The drawing under review shows one solid part. Ordinate dimensions are in mm from its lowest x, y, z. A direction names the side the tool comes from. Round coordinates to 2 decimals unless told otherwise and drop trailing zeros. Order: outer loops, then holes, each group sorted by start corner. A loop starts at its lowest first (then second) coordinate and runs counter-clockwise, first axis right, second up. Notation, with made-up numbers: (14, 16) - (25, 16) arc R30 ccw to (25, 53) - close; hole circle Ø3 at (22.5, 33.5). An arc over 180 degrees is marked (long way). One line per question, with ' | ' between items.
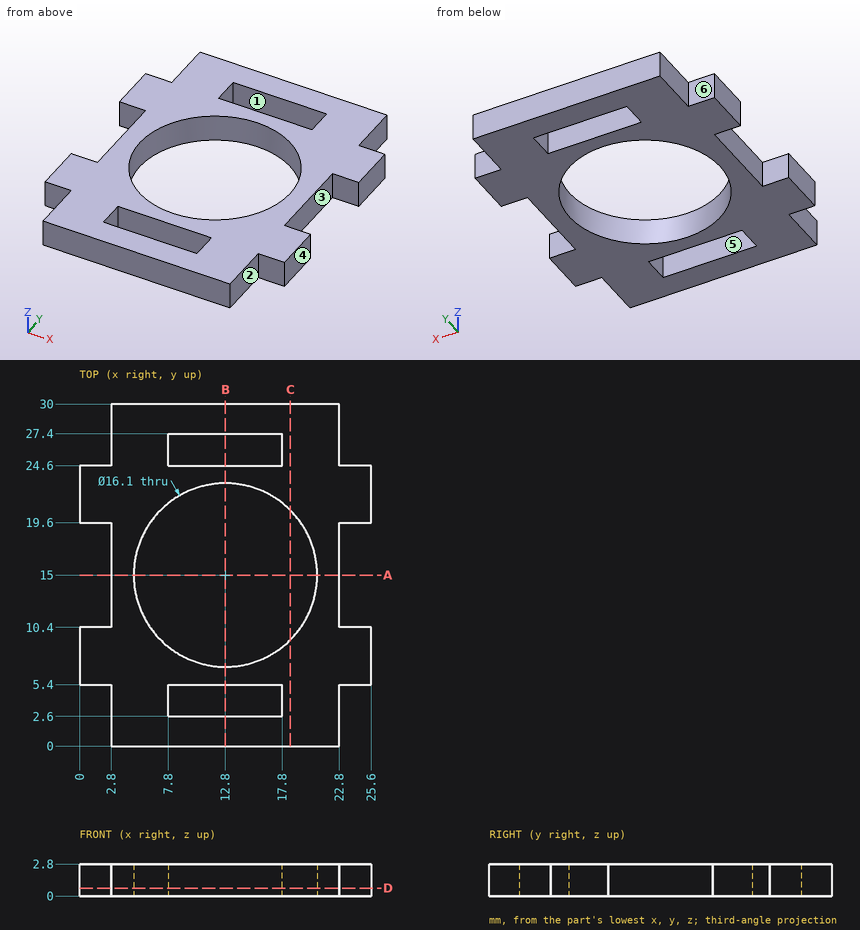
(1) We need section D-D on z = 0.7. Give the number of separate pieces and of enclosed holes in the cut face, plus the area to 3 significant figures.
Output values:
separate pieces: 1 | enclosed holes: 3 | area: 396 mm^2
(2) We need section B-B on x = 12.8. State the section outline as (y, z) points.
Output values:
outline: (0, 0) - (2.6, 0) - (2.6, 2.8) - (0, 2.8) - close; (5.4, 0) - (6.95, 0) - (6.95, 2.8) - (5.4, 2.8) - close; (23.05, 0) - (24.6, 0) - (24.6, 2.8) - (23.05, 2.8) - close; (27.4, 0) - (30, 0) - (30, 2.8) - (27.4, 2.8) - close
(3) Mouldability with a two-part tool opening along X and no side actions: class the marked faces 4, 5 and 6 as released by +X, released by -X, zero draft, split by the parting line, or undercut.
Output values:
face 4: released by +X | face 5: undercut | face 6: zero draft
(4) For the marked faces 1, 2 and 3, list the 3-axis set-ups (+Z, -Z, +X, -X, +Y, -Y) from which the entire face can be reached by the end or side of a thin tool; tool diameter is ignored.
Output values:
face 1: +Z, -Z | face 2: +Z, -Z, +X, -Y | face 3: +Z, -Z, +X
(5) We need section C-C on x = 18.5. State the section outline as (y, z) points, plus the area to 3 significant figures.
Output values:
outline: (0, 0) - (9.32, 0) - (9.32, 2.8) - (0, 2.8) - close; (20.68, 0) - (30, 0) - (30, 2.8) - (20.68, 2.8) - close | area: 52.2 mm^2
(6) Insertion check: pin 1 (6 mm diameter, centred on x = 21, y = 4, fed in from -Z); pin 2 (1.4 mm diameter, centred on y = 3, z = 1, fed in from +X); pin 3 (1.4 mm diameter, centred on y = 4, z = 1, fed in from -X); pin 4 (0.8 mm diameter, centred on x = 1.5, z = 1.5, fed in from -Y). Each pin has a flat end and moves straight along its axis. Give the tip position at first contact, or say it passes through.
Output values:
pin 1: z = 0 | pin 2: x = 22.8 | pin 3: x = 2.8 | pin 4: y = 5.4
(7) For probe 1 along Y at (x, z) = (12.8, 0.9); probe 2 along X at (y, z) = (27, 1.65); probe 3 along X at (y, z) = (2.25, 2.5), list the stretches that pass through material, from the lowest coordinate up. Write a range as [from, to].
Output values:
probe 1: [0, 2.6], [5.4, 6.95], [23.05, 24.6], [27.4, 30] | probe 2: [2.8, 7.8], [17.8, 22.8] | probe 3: [2.8, 22.8]
(8) We need section A-A on y = 15. State the section outline as (x, z) points, plus the area to 3 significant figures.
Output values:
outline: (2.8, 0) - (4.75, 0) - (4.75, 2.8) - (2.8, 2.8) - close; (20.85, 0) - (22.8, 0) - (22.8, 2.8) - (20.85, 2.8) - close | area: 10.9 mm^2
